Verification items for this drawing (mm, ordinates from the low corner). Round coordinates to 2 decimals unless told otherwise and drop trailing zeros. Loops run counter-clockwise (first coordinate to the right, second up) from the corner with the lowest first, then second, coordinate; pieces in that order, holes last. Notation, with made-up numbers: (-15.5, 86) - (11.5, 86) arc R21 cw to (11.5, 95) - close; hole circle Ø4 at (0.5, 57). An arc over 180 degrees is marked (long way). Use a Markdown table: item, result. Add a question column.
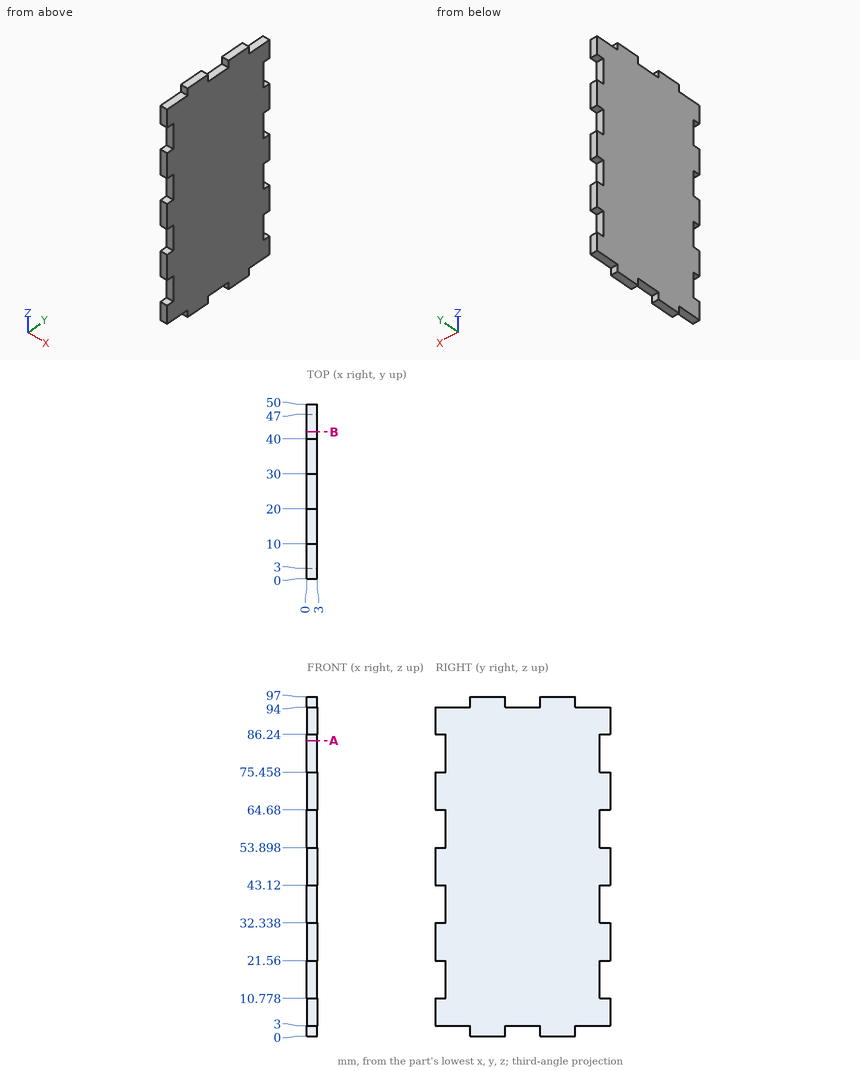
Q1. Section check B-B on y = 42. Record the cut outline in (x, z).
Q2. Thickness scan on line 1 along Y through (x, z) = (1.3, 85.5); line 2 along Z through (x, y) = (1.1, 27). Record the ranges inside material, lowest first.
Q3. Go/stop test with flat-tipped pins: pin 1 Ø0.9 at (x, y) = (2, 49) entering from -Z; pin 2 Ø4 at (y, z) = (5.5, 26) entering from -X; pin 3 Ø0.9 at (x, y) = (1.5, 48.5) entering from +Z. Record where each tip stops, or that it passes through.
Q4. Section check A-A on z = 84.5. Record the cut outline in (x, y), plus the area to 3 significant figures.
Determined:
| question | item | result |
|---|---|---|
| 1 | outline | (0, 3) - (3, 3) - (3, 94) - (0, 94) - close |
| 2 | line 1 | y = 3 to 47 |
| 2 | line 2 | z = 3 to 94 |
| 3 | pin 1 | stops at z = 3 |
| 3 | pin 2 | stops at x = 0 |
| 3 | pin 3 | stops at z = 94 |
| 4 | outline | (0, 3) - (3, 3) - (3, 47) - (0, 47) - close |
| 4 | area | 132 mm² |
